```python
from build123d import *

# Parameters (mm, degrees)
F1_DEPTH      = 25
F1_DEPTH_BACK = 25


with BuildPart() as f1:
    # F0 (on Front) → F1 (new body, two sides)
    with BuildSketch(Plane.XZ) as f1_sk:
        with BuildLine():
            Line((100, 0), (0, 0))
            Line((0, 0), (0, -20))
            Line((0, -20), (100, -20))
            ThreePointArc((100, -20), (121.213203, -28.786797), (130, -50))
            Line((130, -50), (130, -430))
            Line((130, -430), (150, -430))
            Line((150, -430), (150, -50))
            ThreePointArc((150, -50), (135.355339, -14.644661), (100, 0))
        make_face()
    extrude(amount=F1_DEPTH)
    extrude(f1_sk.sketch, amount=-F1_DEPTH_BACK)


solid = f1.part
```
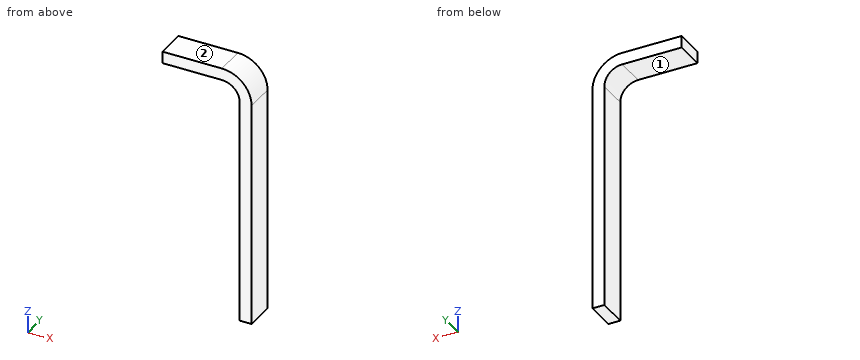
Here's how the part is built. I have some questions about the finished solid (model axes, mm). Face numbers are marked on the shaded views. A direction names the side the tool comes from. Round coordinates to 2 decimals unless told otherwise and drop trailing zeros. Loops run counter-clockwise (first coordinate to the right, second up) from the corner with the lowest first, then second, coordinate; pieces in that order, holes last. Notation, with made-up numbers: (65.25, -21) -> (77.25, -21) arc R31 cw to (77.25, 5) -> close; hole circle Ø10 at (-31, 47.5). An arc over 180 degrees is marked (long way). Answer as CSV lines item,"result". Start each with the question number.
1. I need wall thicknesses on probe 1 along Z at (x, y) = (71, 9); probe 2 along X at (y, z) = (4, -49); probe 3 along Z at (x, y) = (123.5, -21). Which ranges of each line are inside material? Lowest first, please. Write a range as from..to.
2. Imagine slicing it at A-A on y = -2.5. Write out the boundary of the cut face in (x, z), plus the area to 3 significant figures.
3. Imagine slicing it at B-B on z = -174. Write out the boundary of the cut face in (x, y).
4. Imagine slicing it at C-C on x = 54. Write out the boundary of the cut face in (y, z).
5. I'm going to push flat-ended pins straight in: P1, Ø1, axis at y = -11.5, z = -76.5, coming from the -X side; P2, Ø12, axis at x = 51, y = -5, coming from the -Z side; P3, Ø1.5, axis at x = 126, y = 10, coming from the +Z side. Where does each tip first touch, or does it pass through?
6. For the marked faces 1 and 2, which set-ups out of +Z, -Z, +X, -X, +Y, -Y let a thin tool reach every point of the face, with its end or its side?
Solution:
1,probe 1,"-20..0"
1,probe 2,"129.98..149.99"
1,probe 3,"-31.35..-5.87"
2,outline,"(0, -20) -> (100, -20) arc R30 cw to (130, -50) -> (130, -430) -> (150, -430) -> (150, -50) arc R50 ccw to (100, 0) -> (0, 0) -> close"
2,area,"10,900 mm²"
3,outline,"(130, -25) -> (150, -25) -> (150, 25) -> (130, 25) -> close"
4,outline,"(-25, -20) -> (25, -20) -> (25, 0) -> (-25, 0) -> close"
5,P1,"x = 130"
5,P2,"z = -20"
5,P3,"z = -6.84"
6,face 1,"-Z, -X, +Y, -Y"
6,face 2,"+Z, +X, -X, +Y, -Y"
